from build123d import *

# Parameters (mm, degrees)
SKETCH2_R          = 10
SKETCH2_R_2        = 5
CUT_EXTRUDE1_DEPTH = 42


with BuildPart() as part:
    # Sketch1 → Revolve1 (revolve)
    with BuildSketch(Plane.XY):
        Polygon((0, 0), (0, 16), (12, 18), (12, 35), (3, 38), (3, 43), (38, 43), (38, 38), (29, 35), (29, 18), (41, 16), (41, 0), align=None)
    revolve(axis=Axis((0, 0, 0), (1, 0, 0)))

    # Sketch2 → Cut-Extrude1 (cut, through all)
    with BuildSketch(Plane.ZY):
        Circle(SKETCH2_R)
        with Locations((0, 26.5)):
            Circle(SKETCH2_R_2)
        with Locations((26.5, 0)):
            Circle(SKETCH2_R_2)
        with Locations((0, -26.5)):
            Circle(SKETCH2_R_2)
        with Locations((-26.5, 0)):
            Circle(SKETCH2_R_2)
    extrude(amount=-CUT_EXTRUDE1_DEPTH, mode=Mode.SUBTRACT)


solid = part.part
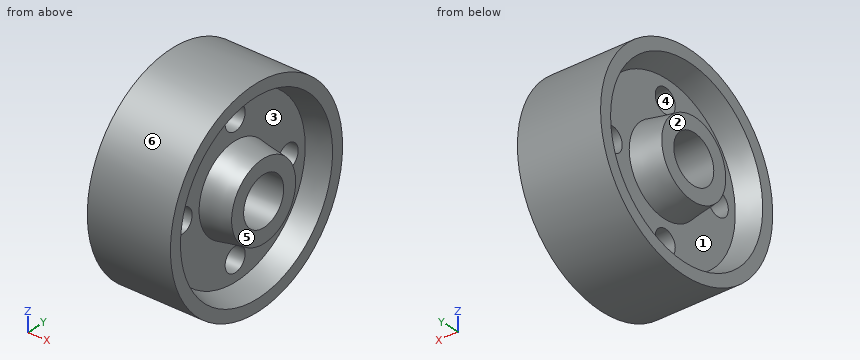
Design review of the part built by this model. Coordinates are the model's own, in mm. Face numbers are marked on the shaded views. A direction names the side the tool comes from. Coordinates: 2 decimals unless noted, no trailing zeros. Order: outer loops, then holes, each group sorted by start corner. A loop starts at its lowest first (then second) coordinate and runs counter-clockwise, first axis right, second up. Notation, with made-up numbers: (58, 28) -> (73, 28) arc R29 cw to (73, 67) -> close; hole circle Ø5 at (-11.5, 44.5). An arc over 180 degrees is marked (long way). Use one line per item in the form item = value. Start each with the question number.
(1) The part is to be moulded in two halves that separate along Z. For the marked faces 4, 5 and 6, say which applies: +Z half, -Z half, draft (parallel to the pull), parting line (faces both ways), or undercut.
(2) Add section A-A on z = 0. Give the number of separate pieces and of enclosed holes in the cut face, plus the area to 3 significant figures.
(3) Insertion check: pin 1 (1 mm diameter, centred on y = -2, z = -28.5, fed in from +X); pin 2 (1.5 mm diameter, centred on x = 7.5, z = -8.5, fed in from +Y); pin 3 (5 mm diameter, centred on x = 26.5, z = -21.5, fed in from -Y); pin 4 (6 mm diameter, centred on x = 13.5, y = -23.5, fed in from -Z). Each pin has a flat end and moves straight along its axis. Give the tip position at first contact, or say it passes through.
(4) For probe 1 along Z at (x, y) = (35, 6); probe 2 along Y at (x, z) = (31, -2.5); probe 3 along Y at (x, z) = (27.5, -1.5), list the stretches that pass through material, from the lowest coordinate up.
(5) Add section C-C on x = 30.5. State the section outline as (y, z) points, plus the area to 3 significant figures.
(6) For the marked faces 1, 2 and 3, list the 3-axis set-ups (+Z, -Z, +X, -X, +Y, -Y) from which the entire face can be reached by the end or side of a thin tool; tool diameter is ignored.
Answer block:
q1.face_4 = undercut
q1.face_5 = draft
q1.face_6 = parting line
q2.separate_pieces = 4
q2.enclosed_holes = 0
q2.area = 1,350 mm²
q3.pin_1 = through
q3.pin_2 = 42.3
q3.pin_3 = -38.57
q3.pin_4 = -37.8
q4.probe_1 = -42.58 to -36.51, -15.91 to -8, 8 to 15.91, 36.51 to 42.58
q4.probe_2 = -42.93 to -35.58, -17.49 to -9.68, 9.68 to 17.49, 35.58 to 42.93
q4.probe_3 = -42.97 to -31.27, -21.73 to -9.89, 9.89 to 21.73, 31.27 to 42.97
q5.outline = circle Ø86 at (0, 0); circle Ø35.5 at (0, 0); hole circle Ø71 at (0, 0); hole circle Ø20 at (0, 0)
q5.area = 2,530 mm²
q6.face_1 = -X
q6.face_2 = +Z, -Z, -X, +Y, -Y
q6.face_3 = +X
